Study the drawing (mm; zero at the part's minimum x, y, z) and answer. Coordinates: 2 decimals unless noted, no trailing zeros. Write each loop counter-clockwise with the first axis right and the second up, starting at its lowest first coordinate (ties: lowest second). Pieces come first, ordered by that corner, then holes. Notation, with made-up numbers: (37.5, -38) - (76.5, -38) arc R7 ccw to (76.5, -28) - close; hole circle Ø10 at (-19, 64.5). An arc over 180 degrees is marked (long way). One line per item, written item: value.
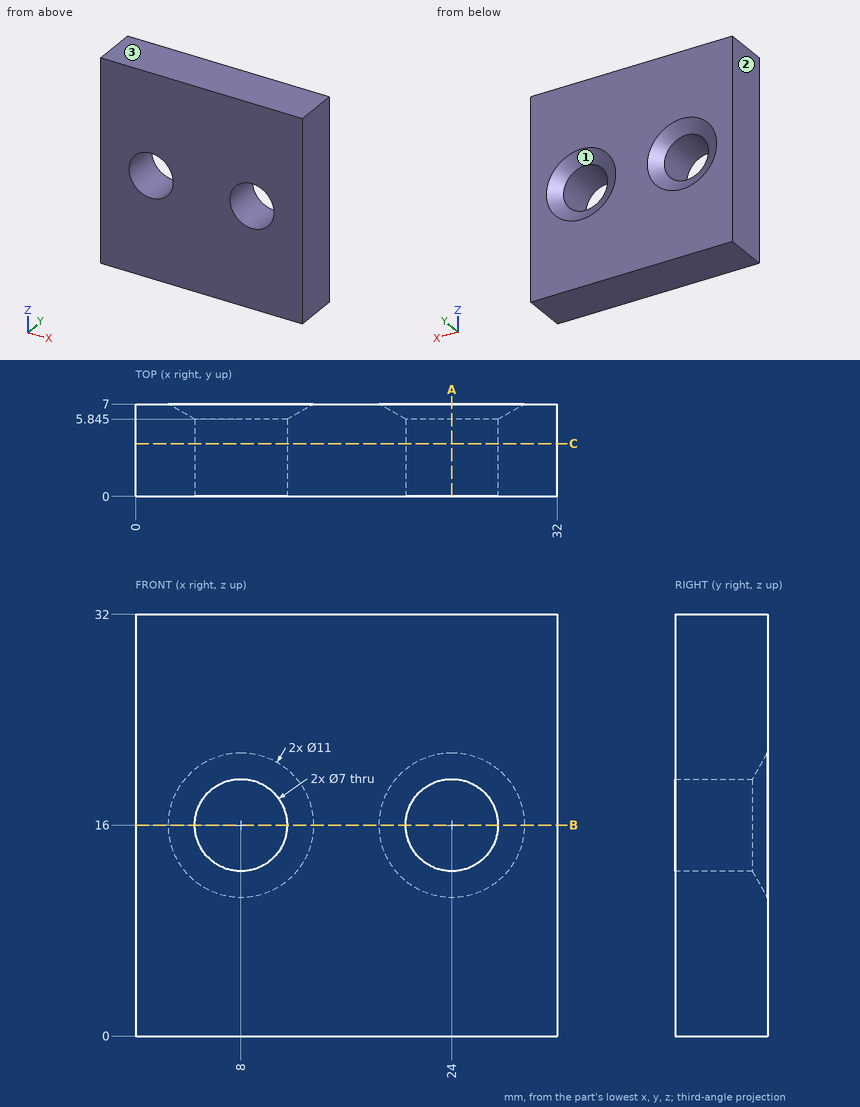
Item 1: Section A-A, the plane x = 24 is taken. Determine the outline of the cut face in (y, z) (1 decimal).
Evaluation:
outline: (0, 0) - (7, 0) - (7, 10.5) - (5.8, 12.5) - (0, 12.5) - close; (0, 19.5) - (5.8, 19.5) - (7, 21.5) - (7, 32) - (0, 32) - close
Item 2: Section B-B, the plane z = 16 is taken. Determine the outline of the cut face in (x, y) (1 decimal).
Evaluation:
outline: (0, 0) - (4.5, 0) - (4.5, 5.8) - (2.5, 7) - (0, 7) - close; (11.5, 0) - (20.5, 0) - (20.5, 5.8) - (18.5, 7) - (13.5, 7) - (11.5, 5.8) - close; (27.5, 0) - (32, 0) - (32, 7) - (29.5, 7) - (27.5, 5.8) - close
Item 3: Determine the mould class of the marked faces 1, 2 and 3 for opening direction Z: +Z half, -Z half, draft (parallel to the pull), parting line (faces both ways), or undercut.
Evaluation:
face 1: undercut
face 2: draft
face 3: +Z half
Item 4: Consider probe 1 along X at (y, z) = (2.1, 16); probe 2 along X at (y, z) = (5.75, 19) (1 decimal); probe 3 along Y at (x, z) = (11.5, 19) (1 decimal). Determine where each line is inside the solid, lowest interval first.
Evaluation:
probe 1: x = 0 to 4.5, 11.5 to 20.5, 27.5 to 32
probe 2: x = 0 to 6.2, 9.8 to 22.2, 25.8 to 32
probe 3: y = 0 to 6.5
Item 5: Section C-C, the plane y = 4 is taken. Determine the outline of the cut face in (x, z).
Evaluation:
outline: (0, 0) - (32, 0) - (32, 32) - (0, 32) - close; hole circle Ø7 at (8, 16); hole circle Ø7 at (24, 16)
